from build123d import *

# Parameters (mm, degrees)
SOLAR_DIVOT_SKETCH_W              = 100
SOLAR_DIVOT_SKETCH_H              = 200
SOLAR_DIVOT_CUT_DEPTH             = 1120
MISC_BAY_SKETCH_W                 = 600
MISC_BAY_SKETCH_H                 = 124.589803375
MISC_BAY_CUT_DEPTH                = 330
LAUNCH_ADAPTOR_BAY_SKETCH_R       = 370
LAUNCH_ADAPTOR_BAY_CUT_DEPTH      = 40
GRIPPER_GAP_CUT_DEPTH             = 100
GRIPPER_GAP_CUT_PROPAGATION_COUNT = 4


with BuildPart() as part:
    # Body Block Sketch → Body Block Revolve (revolve)
    with BuildSketch(Plane.XY, mode=Mode.PRIVATE) as body_block_revolve_sk:
        Polygon((0, 0), (400, 0), (400, 100), (500, 100), (500, 0), (500, -80), (450, -80), (450, -1400), (0, -1400), align=None)
    revolve(body_block_revolve_sk.sketch.rotate(Axis((0, 0, 0), (0, -1, 0)), 180), axis=Axis((0, 0, 0), (0, -1, 0)))

    # Solar Divot Sketch → Solar Divot Cut (cut)
    with BuildSketch(Plane(origin=(0, -180, 0), x_dir=(-1, 0, 0), z_dir=(0, -1, 0))):
        with Locations((-400, 0)):
            Rectangle(SOLAR_DIVOT_SKETCH_W, SOLAR_DIVOT_SKETCH_H)
        with Locations((400, 0)):
            Rectangle(SOLAR_DIVOT_SKETCH_W, SOLAR_DIVOT_SKETCH_H)
    extrude(amount=SOLAR_DIVOT_CUT_DEPTH, mode=Mode.SUBTRACT)

    # Misc Bay Sketch → Misc Bay Cut (cut)
    with BuildSketch(Plane(origin=(0, -180, 0), x_dir=(-1, 0, 0), z_dir=(0, -1, 0))):
        with Locations((0, 387.705098313)):
            Rectangle(MISC_BAY_SKETCH_W, MISC_BAY_SKETCH_H)
        with Locations((0, -387.705098313)):
            Rectangle(MISC_BAY_SKETCH_W, MISC_BAY_SKETCH_H)
    extrude(amount=MISC_BAY_CUT_DEPTH, mode=Mode.SUBTRACT)

    # Launch Adaptor Bay Sketch → Launch Adaptor Bay Cut (cut)
    with BuildSketch(Plane.XZ.offset(1400)):
        Circle(LAUNCH_ADAPTOR_BAY_SKETCH_R)
    extrude(amount=-LAUNCH_ADAPTOR_BAY_CUT_DEPTH, mode=Mode.SUBTRACT)

    # Gripper Gap Sketch → Gripper Gap Cut (cut)
    with BuildSketch(Plane(origin=(0, 0, 0), x_dir=(1, 0, 0), z_dir=(0, 1, 0))):
        Polygon((311.126983722, 395.979797464), (395.979797464, 311.126983722), (42.426406871, -42.426406871), (-42.426406871, 42.426406871), align=None)
    gripper_gap_cut = extrude(amount=GRIPPER_GAP_CUT_DEPTH, mode=Mode.SUBTRACT)

    # Gripper Gap Cut Propagation: Gripper Gap Cut ×4 about axis
    gripper_gap_cut_propagation_axis = Axis((0, 0, 0), (0, 1, 0))
    for i in range(1, GRIPPER_GAP_CUT_PROPAGATION_COUNT):
        add(gripper_gap_cut.rotate(gripper_gap_cut_propagation_axis, i * 360 / GRIPPER_GAP_CUT_PROPAGATION_COUNT), mode=Mode.SUBTRACT)


solid = part.part
CAD build for the part. Positions are in the model's coordinates, mm. A direction names the side the tool comes from. Round coordinates to 2 decimals unless told otherwise and drop trailing zeros. Write each loop counter-clockwise with the first axis right and the second up, starting at its lowest first coordinate (ties: lowest second). Pieces come first, ordered by that corner, then holes.
(1) Slice it at C-C, the plane x = 0. Write the cut outline in (y, z), and give its area (3 significant figures).
(2) Slice it at A-A, the plane z = 0. Write the cut outline in (x, y), and give its area (3 significant figures).
(3) Probe line 1 along Z through (x, y) = (0, -1389); line 2 along Y through (x, z) = (387, 48.5); line 3 along Y through (x, z) = (83.5, 353). List the from-to ranges inside material, lowest first.
(4) Slice it at D-D, the plane x = -419. Write the cut outline in (y, z), and give its area (3 significant figures).
(5) Drop flat-ended pins along their axis: P1, Ø3, axis at y = -826, z = 342.5, coming from the -X side; P2, Ø8, axis at y = -310, z = 332, coming from the -X side; P3, Ø5, axis at y = -399, z = -190.5, coming from the +X side. Give the stop position or say it passes through.
(6) Mould opens along X. For faces 6 (the face through (198.91, -1380.28, 311.985)), 7 (the face through (401, -180, -1)), 8 (the face through (-230.719, 11.26, 443.586)) say: pulls with the +X half, pulls with the -X half, needs draft (parallel to the pull), parting line crosses it, or undercut.
(7) Slice it at B-B, the plane y = -621.5. Write the cut outline in (x, z), and give its area (3 significant figures).
(8) 3-axis set-ups, long thin cutter, end or side, ignore diameter. For faces 1 (the face through (-399, -180, -1)), 2 (the face through (4, -343, -325.41)), 3 (the face through (395, -732, -100)), 4 (the face through (358.247, 49.3, -273.394)), 5 (the face through (4, -343, 325.41)): which of +Z, -Z, +X, -X, +Y, -Y reach the whole face in a straight line?
From the geometry:
1. outline: (-1400, -450) - (-510, -450) - (-510, -325.41) - (-180, -325.41) - (-180, -450) - (-80, -450) - (-80, -500) - (100, -500) - (100, -400) - (0, -400) - (0, 400) - (100, 400) - (100, 500) - (-80, 500) - (-80, 450) - (-180, 450) - (-180, 325.41) - (-510, 325.41) - (-510, 450) - (-1400, 450) - (-1400, 370) - (-1360, 370) - (-1360, -370) - (-1400, -370) - close
1. area: 1,180,000 mm2
2. outline: (-500, -80) - (-450, -80) - (-450, -180) - (-350, -180) - (-350, -1300) - (-450, -1300) - (-450, -1400) - (-370, -1400) - (-370, -1360) - (370, -1360) - (370, -1400) - (450, -1400) - (450, -1300) - (350, -1300) - (350, -180) - (450, -180) - (450, -80) - (500, -80) - (500, 100) - (400, 100) - (400, 0) - (-400, 0) - (-400, 100) - (-500, 100) - close
2. area: 1,030,000 mm2
3. line 1: z = -450 to -370, 370 to 450
3. line 2: y = -1400 to -1300, -180 to 0
3. line 3: y = -1360 to -510, -180 to 0
4. outline: (-1400, -164.13) - (-80, -164.13) - (-80, -272.84) - (100, -272.84) - (100, 272.84) - (-80, 272.84) - (-80, 164.13) - (-1400, 164.13) - close; hole (-1300, -100) - (-180, -100) - (-180, 100) - (-1300, 100) - close
4. area: 308,000 mm2
5. P1: stops at x = -293.63
5. P2: stops at x = -308.08
5. P3: stops at x = 408.85
6. face 6: undercut
6. face 7: needs draft
6. face 8: parting line crosses it
7. outline: (-438.75, -100) arc R450 ccw to (438.75, -100) - (350, -100) - (350, 100) - (438.75, 100) arc R450 ccw to (-438.75, 100) - (-350, 100) - (-350, -100) - close
7. area: 598,000 mm2
8. face 1: -X
8. face 2: -Z
8. face 3: +X
8. face 4: -Z, +Y
8. face 5: +Z
